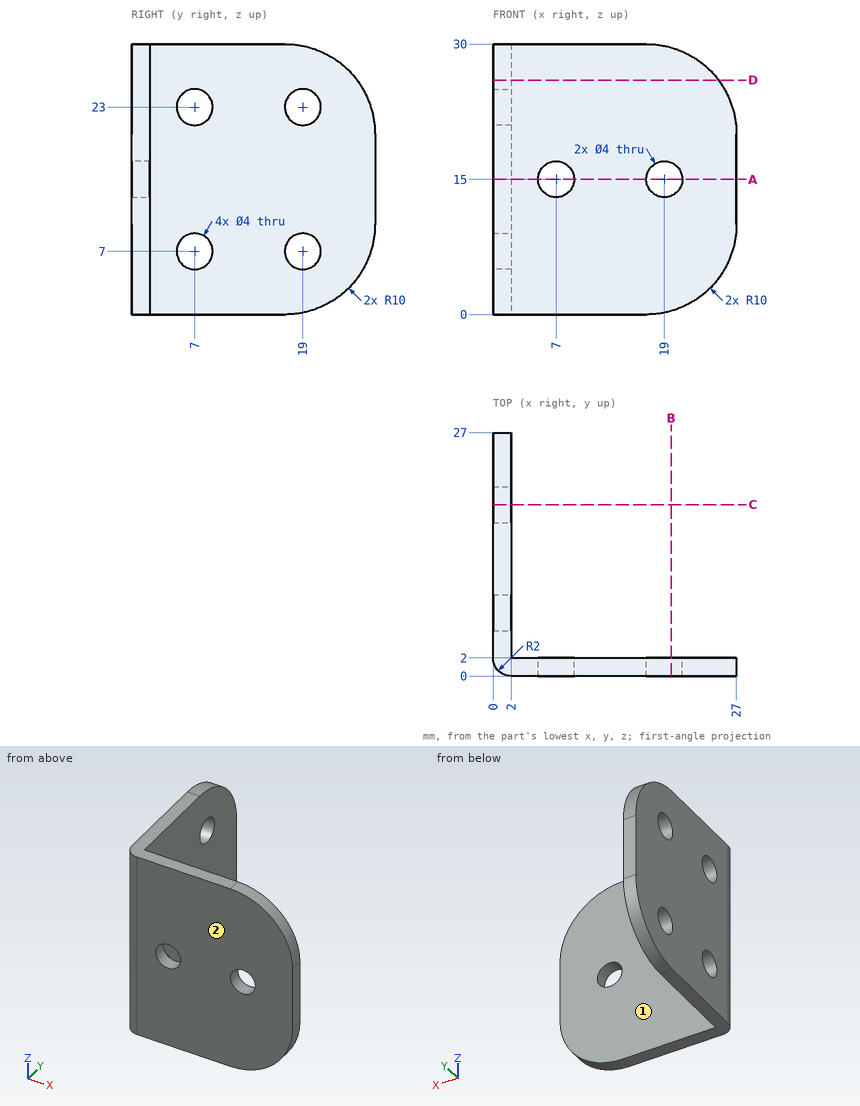
Design review of the part shown in the three views and the two pictorial views. Dimensions are in mm from the part's minimum x, y and z. A direction names the side the tool comes from. Round coordinates to 2 decimals unless told otherwise and drop trailing zeros. Loops run counter-clockwise (first coordinate to the right, second up) from the corner with the lowest first, then second, coordinate; pieces in that order, holes last. Notation, with made-up numbers: M 87,61 L 111,61 A19 ccw 111,92 Z; hole C -8.75,46 d11. An arc over 180 degrees is marked long. Put each result on its own line as item: value.
Q1. Machinability: for the marked faces 1 and 2, which of the approach directions +Z, -Z, +X, -X, +Y, -Y give a long, thin tool a straight path to every point of the face, cutting with its end or side? Answer none if there is none.
Result set:
face 1: +Z, -Z, +X, +Y
face 2: +Z, -Z, +X, -X, -Y
Q2. Consider section C-C, the plane y = 19. Give the boundary of the cut face in (x, z), then the cut area to 3 significant figures.
Result set:
outline: M 0,0.2 L 2,0.2 L 2,5 L 0,5 Z; M 0,9 L 2,9 L 2,21 L 0,21 Z; M 0,25 L 2,25 L 2,29.8 L 0,29.8 Z
area: 43.2 mm²
Q3. To check wall thickness, follow L1, parallel to Y at x = 1.4, z = 7; L2, parallel to X at y = 1.35, z = 15; L3, parallel to Y at x = 4.5, z = 22. State the ranges of each line that lie inside material, in increasing order.
Result set:
L1: y = 0.09 to 5, 9 to 17, 21 to 26.54
L2: x = 0.11 to 5, 9 to 17, 21 to 27
L3: y = 0 to 2
Q4. For pin 1 (2 mm diameter, centred on y = 17.5, z = 4.5, fed in from +X); pin 2 (12 mm diameter, centred on x = 6.5, y = 22, fed in from +Z); pin 3 (4.5 mm diameter, centred on x = 19, z = 15, fed in from +Y), all flat-tipped, find the tip position at first contact; note any pin that passes through.
Result set:
pin 1: stops at x = 2
pin 2: stops at z = 29.95
pin 3: stops at y = 2
Q5. Consider section A-A, the plane z = 15. Give the boundary of the cut face in (x, y), then the cut area to 3 significant figures.
Result set:
outline: M 0,2 A2 ccw 2,0 L 5,0 L 5,2 L 2,2 L 2,27 L 0,27 Z; M 9,0 L 17,0 L 17,2 L 9,2 Z; M 21,0 L 27,0 L 27,2 L 21,2 Z
area: 87.1 mm²
Q6. Consider section D-D, the plane z = 26. Give the boundary of the cut face in (x, y).
Result set:
outline: M 0,2 A2 ccw 2,0 L 25,0 L 25,2 L 2,2 L 2,25 L 0,25 Z
Q7. Consider section B-B, the plane x = 19.75. Give the boundary of the cut face in (y, z), then the cut area to 3 significant figures.
Result set:
outline: M 0,0.39 L 2,0.39 L 2,13.15 L 0,13.15 Z; M 0,16.85 L 2,16.85 L 2,29.61 L 0,29.61 Z
area: 51.0 mm²
